For this review, use the dimensioned drawing (mm, ordinates from the lowest corner) and the shaded views. Coordinates: 2 decimals unless noted, no trailing zeros. Write each loop counter-clockwise with the first axis right and the second up, starting at its lowest first coordinate (ties: lowest second). Pieces come first, ordered by that corner, then holes. Notation, with made-up numbers: M -35.5,85 L 13.5,85 A28 cw 13.5,109 Z; hole C 13,31 d6. An arc over 180 degrees is marked long. One line per question, with ' | ' between items.
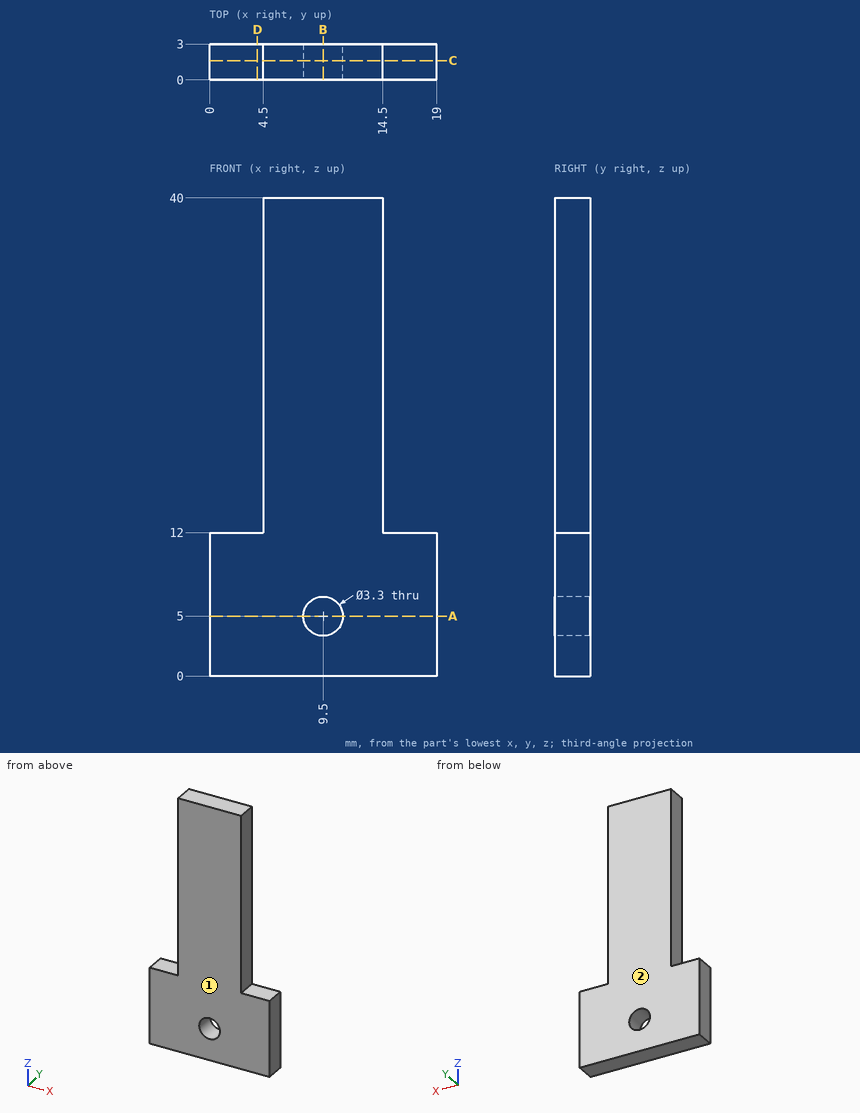
1) We need section D-D on x = 4. State the section outline as (y, z) points, then the cut area to 3 significant figures.
Responses:
outline: M 0,0 L 3,0 L 3,12 L 0,12 Z | area: 36.0 mm^2
2) We need section A-A on z = 5. State the section outline as (x, y) points, then the cut area to 3 significant figures.
Responses:
outline: M 0,0 L 7.85,0 L 7.85,3 L 0,3 Z; M 11.15,0 L 19,0 L 19,3 L 11.15,3 Z | area: 47.1 mm^2
3) Insertion check: pin 1 Ø2.5 at (x, z) = (9.5, 5) entering from -Y; pin 2 Ø1 at (y, z) = (2.5, 24.5) entering from -X; pin 3 Ø1.5 at (x, y) = (16, 2) entering from +Z; pin 4 Ø1 at (y, z) = (1, 21.5) entering from +X. Each pin has a flat end and moves straight along its axis. Give the tip position at first contact, or say it passes through.
Responses:
pin 1: through | pin 2: x = 4.5 | pin 3: z = 12 | pin 4: x = 14.5
4) We need section B-B on x = 9.5. State the section outline as (y, z) points.
Responses:
outline: M 0,0 L 3,0 L 3,3.35 L 0,3.35 Z; M 0,6.65 L 3,6.65 L 3,40 L 0,40 Z
5) The part is to be moulded in two halves that separate along Y. For the marked faces 1 and 2, say which applies: +Y half, -Y half, draft (parallel to the pull), parting line (faces both ways), or undercut.
Responses:
face 1: -Y half | face 2: +Y half
6) To check wall thickness, follow line 1 along X through (y, z) = (1.25, 5); line 2 along Z through (x, y) = (9.5, 1.6); line 3 along X through (y, z) = (2.2, 6). State the ranges of each line that lie inside material, in increasing order. Write a range as [from, to].
Responses:
line 1: [0, 7.85], [11.15, 19] | line 2: [0, 3.35], [6.65, 40] | line 3: [0, 8.19], [10.81, 19]
7) We need section C-C on y = 1.6. State the section outline as (x, z) points, then the cut area to 3 significant figures.
Responses:
outline: M 0,0 L 19,0 L 19,12 L 14.5,12 L 14.5,40 L 4.5,40 L 4.5,12 L 0,12 Z; hole C 9.5,5 d3.3 | area: 499 mm^2
